Geometry: final body of the model. Coordinates: model frame, mm. A direction names the side the tool comes from. Give positions to 0.01 mm unless a question says otherwise; leave off trailing zeros. Loops run counter-clockwise (first coordinate to the right, second up) from the corner with the lowest first, then second, coordinate; pieces in that order, holes last.
1. Section A-A, the plane x = 32.39. Output: boundary loops of the cut face in (y, z).
2. Section B-B, the plane z = -5.75. Output: boundary loops of the cut face in (x, y), then the cut area to 3 significant figures.
3. Access query for faces 4 (the face through (3.65, 0.5, -14.5)), 5 (the face through (18, 0, -8)). Directions: +Z, -Z, +X, -X, +Y, -Y. A direction counts if a zero-diameter tool reaches every point of the face in a straight line with its end or side. Return the directions, or none.
4. Draft query along Z for faces 1 (the face through (8.493, 0.493, -15.462)), 2 (the face through (28, 0.5, -14.5)), 3 (the face through (1.8, 0.5, -16)). Return one class per face: +Z half, -Z half, draft (parallel to the pull), parting line (faces both ways), or undercut.
5. Section D-D, the plane x = 27. Output: boundary loops of the cut face in (y, z), then the cut area to 3 significant figures.
6. Section C-C, the plane y = 0.55. Output: boundary loops of the cut face in (x, z).
7. First-contact query: P1, Ø0.9, axis at x = 16.121, z = -14.613, coming from the -Y side; P2, Ø0.5, axis at x = 5.5, y = 0.5, coming from the -Z side; P3, Ø6, axis at x = 14, z = -9.5, coming from the -Y side. Flat tips, straight axial feed; report the tip coordinate or a pass-through.
8. Material intervals for line 1 along Z through (x, y) = (8.46, 0.7); line 2 along X through (y, z) = (0.7, -6); line 3 along Z through (x, y) = (16, 0.35), sorted ascending.
from build123d import *

# Parameters (mm, degrees)
BOSS_EXTRUDE1_DEPTH     = 1
SKETCH3_R               = 0.75
CUT_EXTRUDE2_DEPTH      = 39.49675311
CUT_EXTRUDE3_DEPTH      = 39.49675311
CUT_EXTRUDE3_DEPTH_BACK = 39.49675311
SKETCH4_R               = 0.75


with BuildPart() as part:
    # Sketch1 → Boss-Extrude1 (new body)
    with BuildSketch(Plane(origin=(0, 0, 0), x_dir=(1, 0, 0), z_dir=(0, 1, 0))):
        Polygon((0, 0), (0, 16), (3.65, 16), (3.65, 12.964), (7.15, 12.964), (7.15, 16), (21.483, 16), (21.483, 12.964), (28, 12.964), (28, 16), (35, 16), (35, 0), align=None)
    extrude(amount=BOSS_EXTRUDE1_DEPTH)

    # Sketch3 → Cut-Extrude2 (cut, through all)
    with BuildSketch(Plane(origin=(0, 1, 0), x_dir=(1, 0, 0), z_dir=(0, 1, 0))):
        with Locations(Location((32.39, 6, 0), (0, 0, 270))):
            Circle(SKETCH3_R)
    extrude(amount=-CUT_EXTRUDE2_DEPTH, mode=Mode.SUBTRACT)

    # Sketch4 → Cut-Extrude3 (cut, two sides: drawn at the far end of the back side and taken through both)
    with BuildSketch(Plane(origin=(0, 1, 0), x_dir=(1, 0, 0), z_dir=(0, 1, 0)).offset(-CUT_EXTRUDE3_DEPTH_BACK)):
        with Locations(Location((8.46, 14.713, 0), (0, 0, 270))):
            Circle(SKETCH4_R)
        with Locations(Location((16.121, 14.613, 0), (0, 0, 270))):
            Circle(SKETCH4_R)
        with Locations(Location((19.121, 14.613, 0), (0, 0, 270))):
            Circle(SKETCH4_R)
    extrude(amount=CUT_EXTRUDE3_DEPTH + CUT_EXTRUDE3_DEPTH_BACK, mode=Mode.SUBTRACT)


solid = part.part
Answers below:
1. outline: (0, -16) - (1, -16) - (1, -6.75) - (0, -6.75) - close; (0, -5.25) - (1, -5.25) - (1, 0) - (0, 0) - close
2. outline: (0, 0) - (31.68, 0) - (31.68, 1) - (0, 1) - close; (33.1, 0) - (35, 0) - (35, 1) - (33.1, 1) - close
2. area: 33.6 mm2
3. face 4: -Z, +Y, -Y
3. face 5: +Z, -Z, +X, -X, -Y
4. face 1: undercut
4. face 2: draft
4. face 3: -Z half
5. outline: (0, -12.96) - (1, -12.96) - (1, 0) - (0, 0) - close
5. area: 13.0 mm2
6. outline: (0, -16) - (3.65, -16) - (3.65, -12.96) - (7.15, -12.96) - (7.15, -16) - (21.48, -16) - (21.48, -12.96) - (28, -12.96) - (28, -16) - (35, -16) - (35, 0) - (0, 0) - close; hole circle Ø1.5 at (8.46, -14.71); hole circle Ø1.5 at (16.12, -14.61); hole circle Ø1.5 at (19.12, -14.61); hole circle Ø1.5 at (32.39, -6)
7. P1: passes through
7. P2: stops at z = -12.96
7. P3: stops at y = 0
8. line 1: z = -16 to -15.46, -13.96 to 0
8. line 2: x = 0 to 31.64, 33.14 to 35
8. line 3: z = -16 to -15.35, -13.87 to 0
